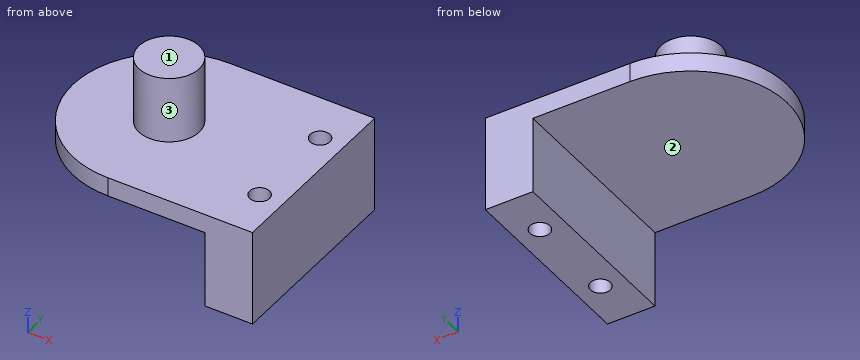
from build123d import *

# Parameters (mm, degrees)
ESQUISSE1_W             = 5
ESQUISSE1_H             = 20.2
BOSS_EXTRU_1_DEPTH      = 8.1
BOSS_EXTRU_2_DEPTH      = 2
ESQUISSE3_R             = 3.175
BOSS_EXTRU_3_DEPTH      = 7
ESQUISSE4_R             = 1.05
ENL_V_MAT_EXTRU_1_DEPTH = 31.236732628


with BuildPart() as part:
    # Esquisse1 → Boss.-Extru.1 (new body)
    with BuildSketch(Plane.XY):
        Rectangle(ESQUISSE1_W, ESQUISSE1_H)
    extrude(amount=BOSS_EXTRU_1_DEPTH)

    # Esquisse2 → Boss.-Extru.2 (add)
    with BuildSketch(Plane.XY.offset(8.1)):
        with BuildLine():
            Line((2.5, 10.1), (-12.7, 10.1))
            ThreePointArc((-12.7, 10.1), (-22.8, 0), (-12.7, -10.1))
            Line((-12.7, -10.1), (2.5, -10.1))
            Line((2.5, -10.1), (2.5, 10.1))
        make_face()
    extrude(amount=BOSS_EXTRU_2_DEPTH)

    # Esquisse3 → Boss.-Extru.3 (add)
    with BuildSketch(Plane.XY.offset(10.1)):
        with Locations((-12.7, 0)):
            Circle(ESQUISSE3_R)
    extrude(amount=BOSS_EXTRU_3_DEPTH)

    # Esquisse4 → Enlèv. mat.-Extru.1 (cut, through all)
    with BuildSketch(Plane(origin=(0, 0, 0), x_dir=(-1, 0, 0), z_dir=(0, 0, -1))):
        with Locations((0, 5)):
            Circle(ESQUISSE4_R)
        with Locations((0, -5)):
            Circle(ESQUISSE4_R)
    extrude(amount=-ENL_V_MAT_EXTRU_1_DEPTH, mode=Mode.SUBTRACT)


solid = part.part
CAD build for the part. Positions are in the model's coordinates, mm. Face numbers are marked on the shaded views. A direction names the side the tool comes from. Give positions to 0.01 mm unless a question says otherwise; leave off trailing zeros. Loops run counter-clockwise (first coordinate to the right, second up) from the corner with the lowest first, then second, coordinate; pieces in that order, holes last. Notation, with made-up numbers: M -23,-24.5 L 10,-24.5 A21 cw 10,-17.5 Z; hole C 9,74 d8. An arc over 180 degrees is marked long. Write each question's results on one line, items separated by ' | '.
Q1. Band-saw the part on C-C on y = 0. Write the cut outline in (x, z) (3 decimals), and give its area (3 significant figures).
Geometry check:
outline: M -22.8,8.1 L -2.5,8.1 L -2.5,0 L 2.5,0 L 2.5,10.1 L -9.525,10.1 L -9.525,17.1 L -15.875,17.1 L -15.875,10.1 L -22.8,10.1 Z | area: 136 mm²
Q2. Flat gauge pins, fed straight in: P1, Ø3, axis at x = -9.5, y = 7.5, coming from the -Z side; P2, Ø2.5, axis at y = -3.5, z = 2.5, coming from the -X side; P3, Ø2.5, axis at x = 0, y = -5, coming from the +Z side; P4, Ø3.5, axis at x = 0, y = 5, coming from the -Z side. Where does each tip first touch, or does it go through?
Geometry check:
P1: stops at z = 8.1 | P2: stops at x = -2.5 | P3: stops at z = 10.1 | P4: stops at z = 0
Q3. Which spindle directions (+Z, -Z, +X, -X, +Y, -Y) get a long thin tool onto all of the face, cutting with end or side? Do the marked faces 1, 2 and 3. Say none if no direction does.
Geometry check:
face 1: +Z, +X, -X, +Y, -Y | face 2: -Z, -X, +Y, -Y | face 3: +Z
Q4. Probe probe 1 along Y at (x, z) = (0, 2.75); probe 2 along Z at (x, y) = (-5.75, -7.25); probe 3 along X at (y, z) = (1.5, 4.75). List the from-to ranges inside material, lowest first.
Geometry check:
probe 1: y = -10.1 to -6.05, -3.95 to 3.95, 6.05 to 10.1 | probe 2: z = 8.1 to 10.1 | probe 3: x = -2.5 to 2.5
Q5. Band-saw the part on D-D on y = 5. Write the cut outline in (x, z).
Geometry check:
outline: M -21.48,8.1 L -2.5,8.1 L -2.5,0 L -1.05,0 L -1.05,10.1 L -21.48,10.1 Z; M 1.05,0 L 2.5,0 L 2.5,10.1 L 1.05,10.1 Z
Q6. Band-saw the part on B-B on z = 6.5. Write the cut outline in (x, y).
Geometry check:
outline: M -2.5,-10.1 L 2.5,-10.1 L 2.5,10.1 L -2.5,10.1 Z; hole C 0,-5 d2.1; hole C 0,5 d2.1
Q7. Band-saw the part on A-A on x = 0. Write the cut outline in (y, z).
Geometry check:
outline: M -10.1,0 L -6.05,0 L -6.05,10.1 L -10.1,10.1 Z; M -3.95,0 L 3.95,0 L 3.95,10.1 L -3.95,10.1 Z; M 6.05,0 L 10.1,0 L 10.1,10.1 L 6.05,10.1 Z
